from build123d import *

# Parameters (mm, degrees)
F0_R     = 3.25
F1_DEPTH = 3


with BuildPart() as f1:
    # F0 (on Top) → F1 (new body)
    with BuildSketch(Plane.XY):
        with BuildLine():
            Line((80.5, 10), (13, 10))
            Line((13, 10), (-10.5, 10))
            ThreePointArc((-10.5, 10), (-12.267767, 9.267767), (-13, 7.5))
            Line((-13, 7.5), (-13, -49.5))
            ThreePointArc((-13, -49.5), (-12.267767, -51.267767), (-10.5, -52))
            Line((-10.5, -52), (10.5, -52))
            ThreePointArc((10.5, -52), (12.267767, -51.267767), (13, -49.5))
            Line((13, -49.5), (13, -12.5))
            ThreePointArc((13, -12.5), (13.732233, -10.732233), (15.5, -10))
            Line((15.5, -10), (80.5, -10))
            ThreePointArc((80.5, -10), (82.267767, -9.267767), (83, -7.5))
            Line((83, -7.5), (83, 7.5))
            ThreePointArc((83, 7.5), (82.267767, 9.267767), (80.5, 10))
        make_face()
        with Locations((0, -12.75)):
            Circle(F0_R, mode=Mode.SUBTRACT)
        with Locations((0, 3.25)):
            Circle(F0_R, mode=Mode.SUBTRACT)
        with Locations((50.435357, 0)):
            Circle(F0_R, mode=Mode.SUBTRACT)
        with Locations((76.45, 0)):
            Circle(F0_R, mode=Mode.SUBTRACT)
    extrude(amount=F1_DEPTH)


solid = f1.part
The listing builds one solid part. Answer for the finished solid, in the listing's coordinates (mm). A direction names the side the tool comes from. Coordinates: 2 decimals unless noted, no trailing zeros. Write each loop counter-clockwise with the first axis right and the second up, starting at its lowest first coordinate (ties: lowest second). Pieces come first, ordered by that corner, then holes. Notation, with made-up numbers: M 11,-12 L 41,-12 A23 ccw 41,19 Z; hole C -39.5,40 d3. An arc over 180 degrees is marked long. Use one line per item in the form item = value.
Item 1: Find section D-D, the plane y = -32. Give the vertices of the cut face in (x, z), plus the area to 3 significant figures.
Model answer:
outline = M -13,0 L 13,0 L 13,3 L -13,3 Z
area = 78.0 mm2
Item 2: Find the intervals of material crossed by probe 1 along Y at (x, z) = (0, 2.2); probe 2 along X at (y, z) = (2, 1.35); probe 3 along X at (y, z) = (-12.5, 2.85), in increasing order.
Model answer:
probe_1 = -52 to -16, -9.5 to 0, 6.5 to 10
probe_2 = -13 to -3, 3 to 47.87, 53 to 73.89, 79.01 to 83
probe_3 = -13 to -3.24, 3.24 to 13
Item 3: For faces 1 (the face through (24, -7, 3)), 2 (the face through (13, -31, 1)), determine the directions among +Z, -Z, +X, -X, +Y, -Y from which every point of the face is accessible in a straight line to the end or side of a thin tool.
Model answer:
face_1 = +Z, +X, -X, +Y, -Y
face_2 = +Z, -Z, +X, -Y
Item 4: Given P1, Ø8.5, axis at x = 0, y = 3.25, coming from the +Z side, flat-ended and moving along its own axis, determine where the tip first touches the part or whether it passes through.
Model answer:
P1 = 3
Item 5: Find section B-B, the plane x = 76.45. Give the vertices of the cut face in (y, z).
Model answer:
outline = M -10,0 L -3.25,0 L -3.25,3 L -10,3 Z; M 3.25,0 L 10,0 L 10,3 L 3.25,3 Z
Item 6: Find section C-C, the plane x = 0. Give the vertices of the cut face in (y, z), plus the area to 3 significant figures.
Model answer:
outline = M -52,0 L -16,0 L -16,3 L -52,3 Z; M -9.5,0 L 0,0 L 0,3 L -9.5,3 Z; M 6.5,0 L 10,0 L 10,3 L 6.5,3 Z
area = 147 mm2
Item 7: The mould has two halves that part along X. Classify faces 3 (the face through (-2.6, 1.3, 1.5)), 4 (the face through (82.248, -9.287, 1.479)), 5 (the face through (0, -52, 1)): released by +X, released by -X, zero draft, split by the parting line, or undercut.
Model answer:
face_3 = undercut
face_4 = released by +X
face_5 = zero draft
Item 8: Find section A-A, the plane z = 2. Give the vertices of the cut face in (x, y).
Model answer:
outline = M -13,-49.5 A2.5 ccw -10.5,-52 L 10.5,-52 A2.5 ccw 13,-49.5 L 13,-12.5 A2.5 cw 15.5,-10 L 80.5,-10 A2.5 ccw 83,-7.5 L 83,7.5 A2.5 ccw 80.5,10 L -10.5,10 A2.5 ccw -13,7.5 Z; hole C 0,-12.75 d6.5; hole C 0,3.25 d6.5; hole C 50.44,0 d6.5; hole C 76.45,0 d6.5
